Can you work these out from the model? Positions are in its coordinate system, mm. A direction names the side the tool comes from. Give positions to 0.01 mm unless a question says otherwise; leave off trailing zeros. Loops run counter-clockwise (first coordinate to the right, second up) from the corner with the lowest first, then second, coordinate; pieces in that order, holes last. Notation, with made-up numbers: (54, -35.5) - (59, -35.5) arc R12 ccw to (59, -25.5) - close; hole circle Ø11 at (84.25, 80). An arc over 180 degrees is marked (long way). Write item = value, one per line.
from build123d import *

# Parameters (mm, degrees)
BOSS_EXTRUDE1_DEPTH            = 25
BOSS_EXTRUDE1_DEPTH_BACK       = 25
CUT_EXTRUDE1_DEPTH             = 103.569488641
CUT_EXTRUDE2_DEPTH             = 103.569488641
F_5_5_5_5_DIAMETER_HOLE1_D     = 5.5
F_5_5_5_5_DIAMETER_HOLE1_DEPTH = 88.997474683
F_5_5_5_5_DIAMETER_HOLE2_D     = 5.5
F_5_5_5_5_DIAMETER_HOLE2_DEPTH = 55.861435714
F_4_2_4_2_DIAMETER_HOLE1_D     = 4.2
FILLET1_R                      = 1.5


with BuildPart() as part:
    # Sketch1 → Boss-Extrude1 (new, two sides: drawn at the far end of the back side and taken through both)
    with BuildSketch(Plane(origin=(7, 0, 0), x_dir=(0, 0, -1), z_dir=(1, 0, 0)).offset(-BOSS_EXTRUDE1_DEPTH_BACK)):
        Polygon((-70, 9), (-70, 0), (0, 0), (49.497474683, 49.497474683), (43.133513652, 55.861435714), (28.991378029, 41.71930009), (-49.991379635, 9), align=None)
    extrude(amount=BOSS_EXTRUDE1_DEPTH + BOSS_EXTRUDE1_DEPTH_BACK)

    # Sketch2 → Cut-Extrude1 (cut, through all)
    with BuildSketch(Plane(origin=(32, 0, 0), x_dir=(0, 0, -1), z_dir=(1, 0, 0))):
        with BuildLine():
            Line((-41.755939666, 5.002860881), (-8.618926871, 5.000000007))
            ThreePointArc((-8.618926871, 5.000000007), (-7.181014363, 6.072472193), (-7.79931621, 7.756364053))
            ThreePointArc((-7.79931621, 7.756364053), (-10.043251633, 11.471008803), (-8.614205769, 15.568771574))
            Line((-8.614205769, 15.568771574), (-10.820032984, 20.895618515))
            Line((-10.820032984, 20.895618515), (-42.237227621, 7.885876783))
            ThreePointArc((-42.237227621, 7.885876783), (-43.142866756, 6.253009411), (-41.755939666, 5.002860881))
        make_face()
    extrude(amount=-CUT_EXTRUDE1_DEPTH, mode=Mode.SUBTRACT)

    # Sketch3 → Cut-Extrude2 (cut, through all)
    with BuildSketch(Plane.ZY.offset(18)):
        with BuildLine():
            Line((-25.924897249, 32.995965061), (-2.558913388, 9.6299812))
            ThreePointArc((-2.558913388, 9.6299812), (-0.788934633, 9.368950353), (-0.028067769, 10.988222878))
            ThreePointArc((-0.028067769, 10.988222878), (1.006237273, 15.208445656), (4.918155981, 17.099730731))
            Line((4.918155981, 17.099730731), (7.125818191, 22.42949878))
            Line((7.125818191, 22.42949878), (-24.290211928, 35.442444531))
            ThreePointArc((-24.290211928, 35.442444531), (-26.111441495, 34.889980582), (-25.924897249, 32.995965061))
        make_face()
    extrude(amount=-CUT_EXTRUDE2_DEPTH, mode=Mode.SUBTRACT)

    # Ø5.5 (5.5) Diameter Hole1
    with Locations(Plane(origin=(0, 0, 0), x_dir=(-1, 0, 0), z_dir=(0, -0.7071067811865477, -0.7071067811865475))):
        with Locations((-7, 59.730322699)):
            Hole(F_5_5_5_5_DIAMETER_HOLE1_D / 2, depth=F_5_5_5_5_DIAMETER_HOLE1_DEPTH)

    # Ø5.5 (5.5) Diameter Hole2
    with Locations(Plane(origin=(0, 0, 0), x_dir=(-1, 0, 0), z_dir=(0, -1, 0))):
        with Locations((-7, -60)):
            Hole(F_5_5_5_5_DIAMETER_HOLE2_D / 2, depth=F_5_5_5_5_DIAMETER_HOLE2_DEPTH)

    # Ø4.2 (4.2) Diameter Hole1 (through all)
    with Locations(Plane.ZY.offset(18)):
        with Locations((4.970562748, 12)):
            Hole(F_4_2_4_2_DIAMETER_HOLE1_D / 2)

    # Fillet1
    fillet1_edges = [part.edges().sort_by_distance(p)[0] for p in [
        (7, 20.895618515, 10.820032984),
        (7, 15.568771574, 8.614205769),
        (7, 22.42949878, 7.125818191),
        (7, 17.099730731, 4.918155981),
    ]]
    fillet(fillet1_edges, radius=FILLET1_R)


solid = part.part
Q1. Imagine slicing it at C-C, the plane z = 60. Write out the boundary of the cut face in (x, y), then the cut area to 4 significant figures.
Output:
outline = (-18, 0) - (4.25, 0) - (4.25, 9) - (-18, 9) - close; (9.75, 0) - (32, 0) - (32, 9) - (9.75, 9) - close
area = 400.5 mm2
Q2. Imagine slicing it at A-A, the plane x = 7. Give the number of separate pieces and of enclosed holes in the cut face, then the cut area to 3 significant figures.
Output:
separate_pieces = 3
enclosed_holes = 3
area = 1,230 mm2
Q3. We'd pull the mould along Z, two halves only. Please class faces 1 (the cylindrical face through (7.35, 12.09, 7.07)), 2 (the flat face through (7, 24, -24)), 3 (the flat face through (7, 0, 35)): released by +Z, released by -Z, zero draft, split by the parting line, or undercut.
Output:
face_1 = undercut
face_2 = released by -Z
face_3 = zero draft
Q4. Imagine slicing it at B-B, the plane y = 25. Write out the boundary of the cut face in (x, z).
Output:
outline = (-18, -25) - (32, -25) - (32, -17.93) - (-18, -17.93) - close; (-18, 0.92) - (32, 0.92) - (32, 11.37) - (-18, 11.37) - close
Q5. For pin 1 (8 mm diameter, centred on y = 27.5, z = 15.5, fed in from +X); pin 2 (9 mm diameter, centred on x = 7, z = 60, fed in from +Y); pin 3 (8 mm diameter, centred on x = -11.5, z = -3, fed in from +Y); pin 4 (4 mm diameter, centred on x = 24.5, y = 49, fed in from -Z), each with a flat end and sliding along its axis, tell me the tip position at first contact or that it passes through.
Output:
pin_1 = 32
pin_2 = 9
pin_3 = 32.61
pin_4 = -49.5
Q6. I need wall thicknesses on L1, parallel to X at y = 5.25, z = 60; L2, parallel to Z at x = 7, y = 6.5; L3, parallel to Y at x = 2, z = 24.5. Which ranges of each line are inside material? Lowest first, please.
Output:
L1 = -18 to 4.25, 9.75 to 32
L2 = -6.5 to 7.12, 43.16 to 57.25, 62.75 to 70
L3 = 0 to 5, 15.23 to 19.56
Q7. Which directions (+Z, -Z, +X, -X, +Y, -Y) give clear straight access to the entire face, cutting with the end or side of a thin tool? Please do faces 4 (the flat face through (32, 18, 6)), 5 (the flat face through (6.65, 19.47, 5.9)).
Output:
face_4 = +Z, -Z, +X, +Y, -Y
face_5 = +X, -X
Q8. Imagine slicing it at D-D, the plane x = -6. Write out the boundary of the cut face in (y, z), then the cut area to 3 significant figures.
Output:
outline = (0, 0) - (49.5, -49.5) - (55.86, -43.13) - (41.72, -28.99) - (9, 49.99) - (9, 70) - (0, 70) - close; hole (5, 8.62) arc R1.5 ccw to (7.76, 7.8) arc R5.1 cw to (14.96, 9.12) arc R1.5 ccw to (16.4, 8.96) - (19.51, 10.25) arc R1.5 ccw to (20.32, 12.21) - (7.89, 42.24) arc R1.5 ccw to (5, 41.76) - close; hole (9.63, -2.56) - (33, -25.92) arc R1.5 ccw to (35.44, -24.29) - (23, 5.74) arc R1.5 ccw to (21.04, 6.55) - (17.93, 5.26) arc R1.5 ccw to (17.03, 4.13) arc R5.1 cw to (10.99, -0.03) arc R1.5 ccw to start; hole circle Ø4.2 at (12, 4.97)
area = 1,330 mm2
